The model under review builds one solid part; all positions refer to its coordinate system, in mm. Face numbers are marked on the shaded views. A direction names the side the tool comes from. Coordinates: 2 decimals unless noted, no trailing zeros. Write each loop counter-clockwise with the first axis right and the second up, starting at its lowest first coordinate (ties: lowest second). Pieces come first, ordered by that corner, then holes.
1) Machinability: for the marked faces 4, 5, 6 and 7, which of the approach directions +Z, -Z, +X, -X, +Y, -Y give a long, thin tool a straight path to every point of the face, cutting with its end or side? Answer none if there is none.
2) Add section B-B, the plane y = 15. State the section outline as (x, z) points.
3) Add section D-D, the plane x = 44. State the section outline as (y, z) points.
4) Mouldability with a two-part tool opening along Z and no side actions: class the marked faces 1, 2 and 3 as released by +Z, released by -Z, zero draft, split by the parting line, or undercut.
5) For line 1 (Y direction, x = 2.2, z = 0); line 2 (Z direction, x = 23, y = -14.5); line 3 (Z direction, x = 66, y = -16.2) (3 decimals), list the stretches that pass through material, from the lowest coordinate up.
6) Add section C-C, the plane z = 15. State the section outline as (x, y) points, then the cut area to 3 significant figures.
7) For P1, Ø10, axis at x = 7.5, z = -27, coming from the +Y side; P2, Ø8, axis at x = 44, y = 0.5, coming from the -Z side; P3, Ø1.5, axis at x = 49, z = -3.5, coming from the -Y side, all flat-tipped, find the tip position at first contact; note any pin that passes through.
8) Add section A-A, the plane z = 0. State the section outline as (x, y) points.
from build123d import *

# Parameters (mm, degrees)
BOSS_EXTRUDE1_DEPTH = 72
SKETCH2_R           = 11.25
SKETCH2_R_2         = 1.75
BOSS_EXTRUDE2_DEPTH = 3
SKETCH3_R           = 1.75
CUT_EXTRUDE1_DEPTH  = 89.386933423


with BuildPart() as part:
    # Sketch1 → Boss-Extrude1 (new body)
    with BuildSketch(Plane(origin=(0, 0, 0), x_dir=(0, 0, -1), z_dir=(1, 0, 0))):
        with BuildLine():
            Line((18.25, 0), (18.25, -18.25))
            Line((18.25, -18.25), (36, -18.25))
            Line((36, -18.25), (36, -15.25))
            Line((36, -15.25), (21.25, -15.25))
            Line((21.25, -15.25), (21.25, 0))
            ThreePointArc((21.25, 0), (0, 21.25), (-21.25, 0))
            Line((-21.25, 0), (-21.25, -15.25))
            Line((-21.25, -15.25), (-36, -15.25))
            Line((-36, -15.25), (-36, -18.25))
            Line((-36, -18.25), (-18.25, -18.25))
            Line((-18.25, -18.25), (-18.25, 0))
            ThreePointArc((-18.25, 0), (0, 18.25), (18.25, 0))
        make_face()
    extrude(amount=BOSS_EXTRUDE1_DEPTH)

    # Sketch2 → Boss-Extrude2 (add)
    with BuildSketch(Plane.ZY):
        with BuildLine():
            Line((-18.25, -18.25), (18.25, -18.25))
            Line((18.25, -18.25), (18.25, 0))
            ThreePointArc((18.25, 0), (0, 18.25), (-18.25, 0))
            Line((-18.25, 0), (-18.25, -18.25))
        make_face()
        Circle(SKETCH2_R, mode=Mode.SUBTRACT)
        with Locations((-15, 0)):
            Circle(SKETCH2_R_2, mode=Mode.SUBTRACT)
        with Locations((0, 15)):
            Circle(SKETCH2_R_2, mode=Mode.SUBTRACT)
        with Locations((15, 0)):
            Circle(SKETCH2_R_2, mode=Mode.SUBTRACT)
        with Locations((0, -15)):
            Circle(SKETCH2_R_2, mode=Mode.SUBTRACT)
    extrude(amount=-BOSS_EXTRUDE2_DEPTH)

    # Sketch3 → Cut-Extrude1 (cut, through all)
    with BuildSketch(Plane(origin=(0, -15.25, 0), x_dir=(1, 0, 0), z_dir=(0, 1, 0))):
        with Locations(Location((36, 28.625, 0), (0, 0, 270))):
            Circle(SKETCH3_R)
        with Locations(Location((6, 28.625, 0), (0, 0, 270))):
            Circle(SKETCH3_R)
        with Locations(Location((66, 28.625, 0), (0, 0, 270))):
            Circle(SKETCH3_R)
        with Locations(Location((66, -28.625, 0), (0, 0, 90))):
            Circle(SKETCH3_R)
        with Locations(Location((36, -28.625, 0), (0, 0, 90))):
            Circle(SKETCH3_R)
        with Locations(Location((6, -28.625, 0), (0, 0, 90))):
            Circle(SKETCH3_R)
    extrude(amount=-CUT_EXTRUDE1_DEPTH, mode=Mode.SUBTRACT)


solid = part.part
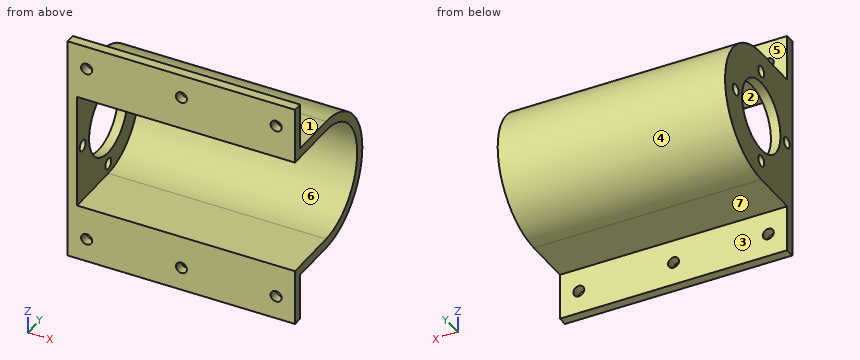
Geometry results:
1. face 4: +X, -X, +Y
1. face 5: +Z, +X, -X, +Y
1. face 6: +X, -Y
1. face 7: -Z, +X, -X, +Y
2. outline: (0, -15.05) - (72, -15.05) - (72, -10.4) - (3, -10.4) - (3, -1.75) - (0, -1.75) - close; (0, 1.75) - (3, 1.75) - (3, 10.4) - (72, 10.4) - (72, 15.05) - (0, 15.05) - close
3. outline: (-18.25, -36) - (-15.25, -36) - (-15.25, -21.25) - (0, -21.25) arc R21.25 ccw to (0, 21.25) - (-15.25, 21.25) - (-15.25, 36) - (-18.25, 36) - (-18.25, 18.25) - (0, 18.25) arc R18.25 cw to (0, -18.25) - (-18.25, -18.25) - close
4. face 1: released by +Z
4. face 2: undercut
4. face 3: zero draft
5. line 1: y = -18.25 to -16.75, -13.25 to -11.25, 11.25 to 13.25, 16.75 to 21.25
5. line 2: z = -21.25 to -18.25, 18.25 to 21.25
5. line 3: z = -36 to -30.375, -26.875 to -18.25, 18.25 to 26.875, 30.375 to 36
6. outline: (0, -18.25) - (3, -18.25) - (3, -1.75) - (0, -1.75) - close; (0, 1.75) - (3, 1.75) - (3, 10.4) - (72, 10.4) - (72, 15.05) - (0, 15.05) - close
6. area: 411 mm2
7. P1: stops at y = -15.25
7. P2: stops at z = -21.25
7. P3: stops at y = 17.75
8. outline: (0, -18.25) - (3, -18.25) - (3, -16.75) - (0, -16.75) - close; (0, -13.25) - (3, -13.25) - (3, -11.25) - (0, -11.25) - close; (0, 11.25) - (3, 11.25) - (3, 13.25) - (0, 13.25) - close; (0, 16.75) - (3, 16.75) - (3, 18.25) - (72, 18.25) - (72, 21.25) - (0, 21.25) - close
